Read the model definition and answer for the solid it produces. Units are mm, in the model's axes. Round coordinates to 2 decimals unless told otherwise and drop trailing zeros. Order: outer loops, then holes, each group sorted by start corner. A loop starts at its lowest first (then second) coordinate and runs counter-clockwise, first axis right, second up. Notation, with made-up numbers: (48, -31) - (84, -31) arc R12 ccw to (84, -22) - close; hole circle Ø6 at (7.5, -15). An arc over 180 degrees is marked (long way). Put each result on its own line as item: value. Start each with the question number.
Q1. Section A-A on x = 316.5 is taken. Give the vertices of the cut face in (y, z), then the cut area to 3 significant figures.
Q2. Section B-B on y = -11.75 is taken. Give the vertices of the cut face in (x, z).
Q3. Each of these flat-tipped pins is pushed along its axis until it touches: pin 1 Ø1 at (x, z) = (-331, 38) entering from -Y; pin 2 Ø8 at (y, z) = (-5.5, 24.5) entering from +X; pin 3 Ø6 at (x, y) = (-316.5, -13.5) entering from +Z. Where does it stop, or does it pass through?
Q4. Section C-C on z = 26 is taken. Give the vertices of the cut face in (x, y).
Q5. Find the intervals of material crossed by line 1 along Y through (x, z) = (510, 8.5); line 2 along Z through (x, y) = (176.5, -7.75); line 3 along Z through (x, y) = (408.5, -16.75), in increasing order. Write a range as from..to.
Q6. For a pull along Z with two mould halves and no side action, classify faces 1 (the face through (8, -1.2, 20)), 2 (the face through (8, -11, 1.2)), 3 (the face through (8, -11, 0)), 4 (the face through (8, 0, 20)) as pulls with the +Z half, pulls with the -Z half, needs draft (parallel to the pull), parting line crosses it, or undercut.
from build123d import *

# Parameters (mm, degrees)
BASE_FLANGE1_DEPTH   = 560
EDGE_FLANGE1_START   = -560
EDGE_FLANGE1_DEPTH   = 1120
EDGE_FLANGE1_2_DEPTH = 1120


# Read off the part's stored shape, not the designer's step: Edge-Flange1
# Sheet-metal steps are written as plain solids
with BuildPart() as part:
    # Sketch1 → Base-Flange1 (new, symmetric)
    with BuildSketch(Plane(origin=(0, 0, 0), x_dir=(0, 0, -1), z_dir=(1, 0, 0))):
        with BuildLine():
            Line((0, -20), (0, -1.9366))
            ThreePointArc((0, -1.9366), (-0.567217008, -0.567217008), (-1.9366, 0))
            Line((-1.9366, 0), (-40, 0))
            Line((-40, 0), (-40, -1.2))
            Line((-40, -1.2), (-1.9366, -1.2))
            ThreePointArc((-1.9366, -1.2), (-1.415745145, -1.415745145), (-1.2, -1.9366))
            Line((-1.2, -1.9366), (-1.2, -20))
            Line((-1.2, -20), (0, -20))
        make_face()
    extrude(amount=BASE_FLANGE1_DEPTH, both=True)

    # Edge-Flange1 outline → Edge-Flange1 (cut)
    with BuildSketch(Plane.YZ.offset(EDGE_FLANGE1_START)):
        with BuildLine():
            Line((-1.2, 40), (-0.567217008, 39.367217008))
            ThreePointArc((-0.567217008, 39.367217008), (-0.147414897, 38.738938751), (0, 37.997834015))
            Line((0, 37.997834015), (0, 40))
            Line((0, 40), (-1.2, 40))
        make_face()
    extrude(amount=EDGE_FLANGE1_DEPTH, mode=Mode.SUBTRACT)

    # Edge-Flange1 2 outline → Edge-Flange1 2 (add)
    with BuildSketch(Plane.YZ.offset(EDGE_FLANGE1_START)):
        with BuildLine():
            Line((-1.2, 37.997834015), (-1.2, 40))
            Line((-1.2, 40), (-7.071067812, 45.871067812))
            Line((-7.071067812, 45.871067812), (-7.919595949, 45.022539674))
            Line((-7.919595949, 45.022539674), (-1.415745145, 38.51868887))
            ThreePointArc((-1.415745145, 38.51868887), (-1.256070336, 38.279718631), (-1.2, 37.997834015))
        make_face()
    extrude(amount=EDGE_FLANGE1_2_DEPTH)


solid = part.part
Findings:
1. outline: (-20, 0) - (-1.94, 0) arc R1.94 ccw to (0, 1.94) - (0, 38) arc R1.94 ccw to (-0.57, 39.37) - (-7.07, 45.87) - (-7.92, 45.02) - (-1.42, 38.52) arc R0.74 cw to (-1.2, 38) - (-1.2, 1.94) arc R0.74 cw to (-1.94, 1.2) - (-20, 1.2) - close
1. area: 79.8 mm2
2. outline: (-560, 0) - (560, 0) - (560, 1.2) - (-560, 1.2) - close
3. pin 1: y = -1.4
3. pin 2: through
3. pin 3: z = 1.2
4. outline: (-560, -1.2) - (560, -1.2) - (560, 0) - (-560, 0) - close
5. line 1: -1.2..0
5. line 2: 0..1.2, 44.85..45.19
5. line 3: 0..1.2
6. face 1: undercut
6. face 2: undercut
6. face 3: pulls with the -Z half
6. face 4: needs draft
